Check sheet for the modelled part. Datum: model origin and axes. Units: mm. Face numbers are marked on the shaded views. A direction names the side the tool comes from. Round coordinates to 2 decimals unless told otherwise and drop trailing zeros. Loops run counter-clockwise (first coordinate to the right, second up) from the corner with the lowest first, then second, coordinate; pieces in that order, holes last. Notation, with made-up numbers: (41, 68.5) -> (50, 68.5) arc R16 ccw to (50, 74.5) -> close; hole circle Ø7 at (46.5, -11). An arc over 180 degrees is marked (long way). Return JSON: item names as keys, results as strings.
from build123d import *

# Parameters (mm, degrees)
BOX_W             = 50
BOX_H             = 37
BOX_DEPTH         = 16
BOX001_W          = 35
BOX001_H          = 35
BOX001_DEPTH      = 20
BOX002_W          = 11
BOX002_H          = 10
BOX002_DEPTH      = 12.5
CYLINDER_R        = 3.35
CYLINDER_DEPTH    = 22
SKETCH_W          = 2
SKETCH_H          = 36
POCKET_DEPTH      = 5
CYLINDER001_R     = 3.35
CYLINDER001_DEPTH = 1
CYLINDER002_R     = 2.8
CYLINDER002_DEPTH = 1
PAD_DEPTH         = 10
PAD001_DEPTH      = 10


with BuildPart() as part:
    # Box → Box (join)
    with BuildSketch(Plane.XY):
        with Locations((25, 18.5)):
            Rectangle(BOX_W, BOX_H)
    extrude(amount=BOX_DEPTH)

    # Box001 → Box001 (cut)
    with BuildSketch(Plane(origin=(1, 1, 2), x_dir=(1, 0, 0), z_dir=(0, 0, 1))):
        with Locations((17.5, 17.5)):
            Rectangle(BOX001_W, BOX001_H)
    extrude(amount=BOX001_DEPTH, mode=Mode.SUBTRACT)

    # Box002 → Box002 (join)
    with BuildSketch(Plane(origin=(39, 6, 16), x_dir=(1, 0, 0), z_dir=(0, 0, 1))):
        with Locations((5.5, 5)):
            Rectangle(BOX002_W, BOX002_H)
    extrude(amount=BOX002_DEPTH)

    # Cylinder → Cylinder (cut)
    with BuildSketch(Plane(origin=(28, 11, 23.5), x_dir=(0, 1, 0), z_dir=(1, 0, 0))):
        Circle(CYLINDER_R)
    extrude(amount=CYLINDER_DEPTH, mode=Mode.SUBTRACT)

    # Sketch (on Sketch) → Pocket (cut)
    with BuildSketch(Plane(origin=(38, 13.1, 2), x_dir=(0, -1, 0), z_dir=(0, 0, 1))):
        with Locations((-19.9, -19)):
            Rectangle(SKETCH_W, SKETCH_H)
        with Locations((-15.9, -19)):
            Rectangle(SKETCH_W, SKETCH_H)
        with Locations((-11.9, -19)):
            Rectangle(SKETCH_W, SKETCH_H)
        with Locations((-7.9, -19)):
            Rectangle(SKETCH_W, SKETCH_H)
        with Locations((-3.9, -19)):
            Rectangle(SKETCH_W, SKETCH_H)
        with Locations((0.1, -19)):
            Rectangle(SKETCH_W, SKETCH_H)
        with Locations((4.1, -19)):
            Rectangle(SKETCH_W, SKETCH_H)
        with Locations((8.1, -19)):
            Rectangle(SKETCH_W, SKETCH_H)
    extrude(amount=-POCKET_DEPTH, mode=Mode.SUBTRACT)

    # Cylinder001 → Cylinder001 (join)
    with BuildSketch(Plane(origin=(39, 11, 23.5), x_dir=(0, -1, 0), z_dir=(1, 0, 0))):
        Circle(CYLINDER001_R)
    extrude(amount=CYLINDER001_DEPTH)

    # Cylinder002 → Cylinder002 (cut)
    with BuildSketch(Plane(origin=(40, 11, 23.5), x_dir=(0, 1, 0), z_dir=(-1, 0, 0))):
        Circle(CYLINDER002_R)
    extrude(amount=CYLINDER002_DEPTH, mode=Mode.SUBTRACT)

    # Sketch002 (on Face11 of Cylinder002) → Pad (join)
    with BuildSketch(Plane(origin=(34, 11, 23.5), x_dir=(0, 1, 0), z_dir=(-1, 0, 0))):
        Polygon((-10, 7.5), (-9, 7.5), (-10, 8.5), align=None)
    extrude(amount=PAD_DEPTH)

    # Sketch003 (on Face10 of Pad) → Pad001 (join)
    with BuildSketch(Plane(origin=(40, 3, 23.5), x_dir=(0, 0, -1), z_dir=(0, 1, 0))):
        Polygon((7.5, 4), (7.5, 5), (8.5, 4), align=None)
    extrude(amount=PAD001_DEPTH)


solid = part.part
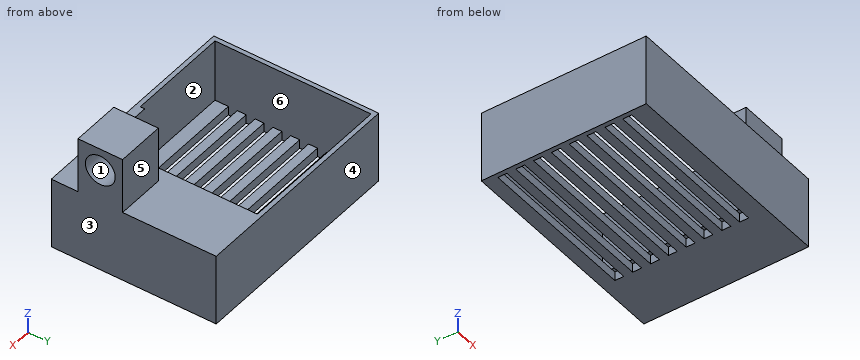
Q1. Section check B-B (y = 33). Record the boundary of the cut face in (x, z).
Results list:
{"outline": "(0, 0) -> (1, 0) -> (1, 16) -> (0, 16) -> close; (36, 2) -> (37, 2) -> (37, 0) -> (50, 0) -> (50, 16) -> (36, 16) -> close"}
Q2. Go/stop test with flat-tipped pins: pin 1 (1 mm diameter, centred on x = 31.5, y = 7, fed in from +Z); pin 2 (1.5 mm diameter, centred on y = 12.5, z = 13, fed in from -X); pin 3 (6 mm diameter, centred on x = 34.5, y = 21, fed in from +Z); pin 4 (0.5 mm diameter, centred on x = 36.5, y = 17, fed in from -Z). Record where each tip stops, or that it passes through.
Results list:
{"pin 1": "z = 2", "pin 2": "x = 0", "pin 3": "z = 16", "pin 4": "z = 2"}
Q3. Section check A-A (z = 23.5). Record the boundary of the cut face in (x, y), then the cut area to 3 significant figures.
Results list:
{"outline": "(39, 6) -> (50, 6) -> (50, 7.65) -> (40, 7.65) -> (40, 8.2) -> (39, 8.2) -> close; (39, 13.8) -> (40, 13.8) -> (40, 14.35) -> (50, 14.35) -> (50, 16) -> (39, 16) -> close", "area": "37.4 mm^2"}
Q4. Material ranges on line 1 (X direction, y = 7, z = 9.5); line 2 (Y direction, x = 39.8, z = 23.5); line 3 (Y direction, x = 44.25, z = 23.5), recorded low to high.
Results list:
{"line 1": "0 to 1, 36 to 50", "line 2": "6 to 8.2, 13.8 to 16", "line 3": "6 to 7.65, 14.35 to 16"}
Q5. Draft check along X on the marked faces 1, 2 and 3. Enter one of: released by +X, released by -X, zero draft, split by the parting line, or undercut.
Results list:
{"face 1": "zero draft", "face 2": "undercut", "face 3": "released by +X"}
Q6. Tool access check on the marked faces 4, 5 and 6. Record the directions out of +Z, -Z, +X, -X, +Y, -Y that give a thin tool (end or side, any length) a straight path to the whole face; none if there is none.
Results list:
{"face 4": "+Z, -Z, +X, -X, +Y", "face 5": "+Z, +X, -X, +Y", "face 6": "+Z"}
Q7. Section check D-D (z = 10.75). Record the boundary of the cut face in (x, y), then the cut area to 3 significant figures.
Results list:
{"outline": "(0, 0) -> (50, 0) -> (50, 37) -> (0, 37) -> close; hole (1, 1) -> (36, 1) -> (36, 36) -> (1, 36) -> close", "area": "625 mm^2"}
Q8. Section check C-C (x = 41). Record the boundary of the cut face in (y, z), then the cut area to 3 significant figures.
Results list:
{"outline": "(0, 0) -> (37, 0) -> (37, 16) -> (16, 16) -> (16, 28.5) -> (6, 28.5) -> (6, 16) -> (0, 16) -> close; hole circle Ø6.7 at (11, 23.5)", "area": "682 mm^2"}
